The listing builds one solid part. Answer for the finished solid, in the listing's coordinates (mm). Round coordinates to 2 decimals unless told otherwise and drop trailing zeros. Write each loop counter-clockwise with the first axis right and the second up, starting at its lowest first coordinate (ties: lowest second). Pieces come first, ordered by that corner, then holes. Notation, with made-up numbers: (71, 82.25) - (123, 82.25) arc R14 cw to (123, 89.25) - close; hole circle Ø8 at (31.25, 16.5). An arc over 180 degrees is marked (long way). Return JSON: item names as keys, results as strings. Group by question number.
Autodesk Inventor part; units mm, degrees
ref_plane "YZ Plane" through (0, 0, 0) normal (1, 0, 0) x (0, 1, 0)
ref_plane "XZ Plane" through (0, 0, 0) normal (0, 1, 0) x (-1, 0, 0)
ref_plane "XY Plane" through (0, 0, 0) normal (0, 0, 1) x (1, 0, 0)
sketch "Sketch1" plane through (0, 0, 0) normal (0, 1, 0) x (-1, 0, 0)
  line L0 (-548.1175, 185.8202) -> (-328.9504, 143.2184)
  line L1 (-547.9214, -184.3469) -> (-328.7026, -141.7351)
  arc A0 (-547.9214, -184.3469) -> (-548.1175, 185.8202) centre (-2.1062, 1.0257) ccw
  arc A1 (-328.7026, -141.7351) -> (-328.9504, 143.2184) centre (-2.1062, 1.0257) ccw
  circle A2 centre (-340.5404, 165.8456) radius 10
  circle A3 centre (-521.3675, 200.9948) radius 10
  line L2 (-296.1915, 1.3356) -> (-698.7298, 1.3356)
  circle A4 centre (-340.5404, -163.1743) radius 10
  circle A5 centre (-521.3675, -198.3235) radius 10
  circle A6 centre (376.435, 0) radius 10
  circle A7 centre (556.435, 0) radius 10
  circle A8 centre (58.8874, 371.8005) radius 10
  circle A9 centre (87.0456, 549.5844) radius 10
  circle A10 centre (58.8874, -371.8005) radius 10
  circle A11 centre (87.0456, -549.5844) radius 10
  point P0 (0, 0)
  dimension "d34" = 1152.87
  dimension "d48" = 712.87
  dimension "d52" = 20
  dimension "d53" = 20
  dimension "d54" = 376.435
  dimension "d55" = 20
  dimension "d56" = 20
  dimension "d58" = 556.435
  dimension "d59" = 20
  dimension "d60" = 376.435
  dimension "d61" = 20
  dimension "d62" = 556.435
  dimension "d65" = 81
  dimension "d69" = 81
extrude "Extrusion1" add sketch "Sketch1" along normal blind 7
properties part number "Shelf"
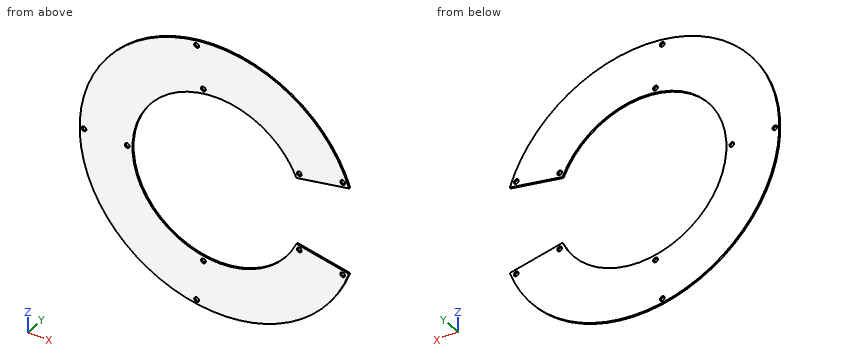
(1) Find section D-D (z = 42). Write down the section's boundary in (x, y), plus the area to 3 significant figures.
(2) Find section C-C (y = 3.5). State how many separate pieces and enclosed holes the cut face has, plus the area to 3 significant figures.
(3) Find section B-B (z = -336.5). Write down the section's boundary in (x, y), plus the area to 3 significant figures.
(4) Consider line 1 (Z direction, x = 241, y = 0.5); line 2 (Z direction, x = 452, y = 4); line 3 (X direction, y = 0.5, z = -211). Determine where each line is inside the solid, lowest interval first.
(5) Find section A-A (x = 201.5). Write down the section's boundary in (y, z), plus the area to 3 significant figures.
(6) Flat-ended cylindrical pins translate along their axes: pin 1 (1 mm diameter, centred on x = -238.5, y = 3, fed in from -Z); pin 2 (1.5 mm diameter, centred on y = 3.5, z = -455, fed in from -X); pin 3 (3 mm diameter, centred on x = 324, y = 5, fed in from -Z); pin 4 (18 mm diameter, centred on x = 521.37, z = -198.32, fed in from -Y). Find the tip coordinate at first contact, or state that the pin passes through.
Check sheet entries:
{
 "1": {"outline": "(-572.87, 0) - (-351.97, 0) - (-351.97, 7) - (-572.87, 7) - close", "area": "1,550 mm^2"},
 "2": {"separate pieces": "1", "enclosed holes": "10", "area": "568,000 mm^2"},
 "3": {"outline": "(-465.18, 0) - (-112.45, 0) - (-112.45, 7) - (-465.18, 7) - close; (116.66, 0) - (469.39, 0) - (469.39, 7) - (116.66, 7) - close", "area": "4,940 mm^2"},
 "4": {"line 1": "z = -523.58 to -263.5, 265.55 to 525.63", "line 2": "z = -359.35 to -165.7, 167.14 to 361.4", "line 3": "x = -533.92 to -284.41, 288.62 to 538.13"},
 "5": {"outline": "(0, -539.82) - (7, -539.82) - (7, -294.42) - (0, -294.42) - close; (0, 296.47) - (7, 296.47) - (7, 541.88) - (0, 541.88) - close", "area": "3,440 mm^2"},
 "6": {"pin 1": "stops at z = -523.02", "pin 2": "stops at x = -351.45", "pin 3": "stops at z = -478.17", "pin 4": "passes through"}
}
